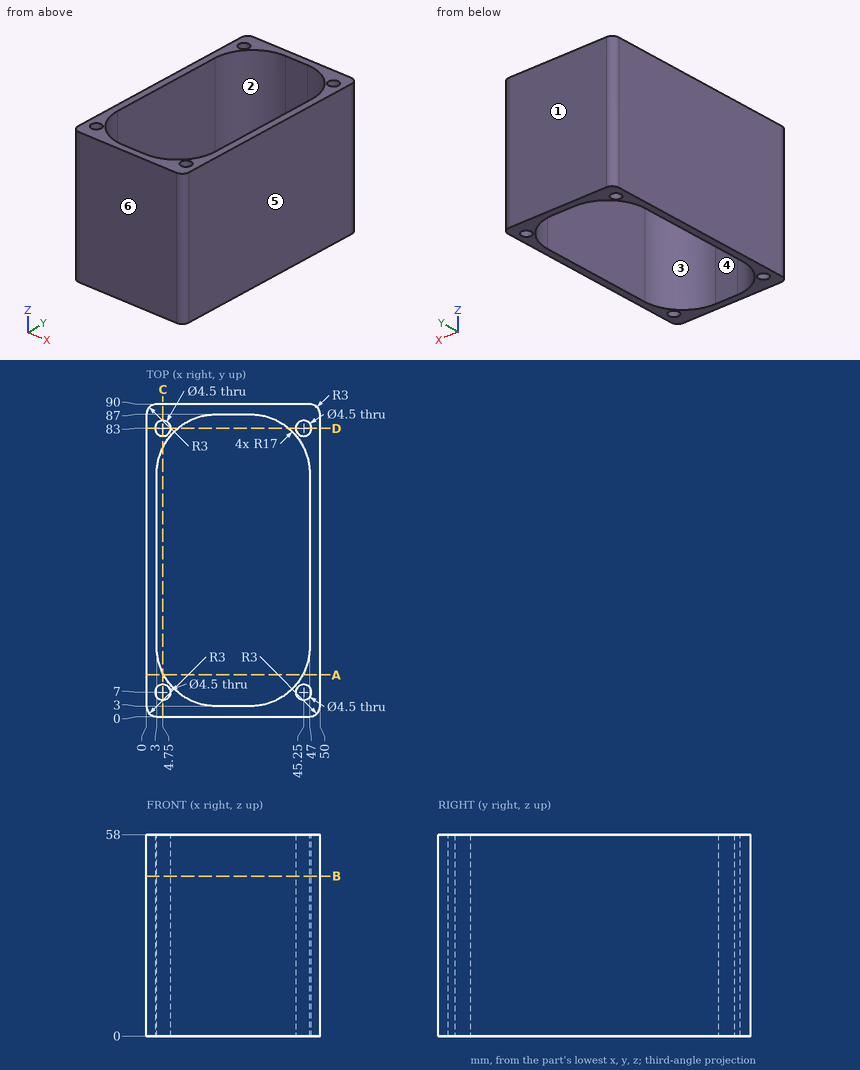
Geometry check sheet. Reference: drawing and pictorial views, mm from the part's lowest x, y, z. A direction names the side the tool comes from. Coordinates: 2 decimals unless noted, no trailing zeros. Order: outer loops, then holes, each group sorted by start corner. A loop starts at its lowest first (then second) coordinate and runs counter-clockwise, first axis right, second up. Notation, with made-up numbers: (63.25, 43) - (85.25, 43) arc R18 cw to (85.25, 66) - close; hole circle Ø9 at (9.5, 29). An arc over 180 degrees is marked (long way). One line per item, written item: value.
(1) Sectioned sample at B-B (z = 46). Enter the section's corners in (x, y), and give its area (3 significant figures).
Data:
outline: (0, 3) arc R3 ccw to (3, 0) - (47, 0) arc R3 ccw to (50, 3) - (50, 87) arc R3 ccw to (47, 90) - (3, 90) arc R3 ccw to (0, 87) - close; hole circle Ø4.5 at (4.75, 7); hole circle Ø4.5 at (4.75, 83); hole (3, 20) arc R17 ccw to (20, 3) - (30, 3) arc R17 ccw to (47, 20) - (47, 70) arc R17 ccw to (30, 87) - (20, 87) arc R17 ccw to (3, 70) - close; hole circle Ø4.5 at (45.25, 7); hole circle Ø4.5 at (45.25, 83)
area: 981 mm^2
(2) Sectioned sample at C-C (x = 4.75). Enter the section's corners in (y, z).
Data:
outline: (0, 0) - (4.75, 0) - (4.75, 58) - (0, 58) - close; (9.25, 0) - (12.49, 0) - (12.49, 58) - (9.25, 58) - close; (77.51, 0) - (80.75, 0) - (80.75, 58) - (77.51, 58) - close; (85.25, 0) - (90, 0) - (90, 58) - (85.25, 58) - close
(3) Release check for a two-part mould opening along Y. For the marked faces 3, 4, 5 and 6 record: +Y half, -Y half, draft (parallel to the pull), parting line (faces both ways), or undercut.
Data:
face 3: undercut
face 4: undercut
face 5: draft
face 6: -Y half
(4) Access from +Z, -Z, +X, -X, +Y, -Y to the whole of each face (thin tool, end or side, straight path). Record for the marked faces 1 and 2.
Data:
face 1: +Z, -Z, +X, -X, +Y
face 2: +Z, -Z
(5) Sectioned sample at A-A (y = 12). Enter the section's corners in (x, z).
Data:
outline: (0, 0) - (5, 0) - (5, 58) - (0, 58) - close; (45, 0) - (50, 0) - (50, 58) - (45, 58) - close
(6) Depth check by flat-ended pin: pin 1 Ø5 at (y, z) = (24, 50.5) entering from -X; pin 2 Ø4 at (x, y) = (8, 77) entering from +Z. Enter the tip coordinate at first touch or a pass-through.
Data:
pin 1: stops at x = 0
pin 2: passes through
(7) Sectioned sample at D-D (y = 83). Enter the section's corners in (x, z), and give its area (3 significant figures).
Data:
outline: (0, 0) - (2.5, 0) - (2.5, 58) - (0, 58) - close; (7, 0) - (9.05, 0) - (9.05, 58) - (7, 58) - close; (40.95, 0) - (43, 0) - (43, 58) - (40.95, 58) - close; (47.5, 0) - (50, 0) - (50, 58) - (47.5, 58) - close
area: 527 mm^2
(8) Thickness scan on probe 1 along X at (y, z) = (57, 18.5); probe 2 along X at (y, z) = (5, 29); probe 3 along Y at (x, z) = (4.75, 33.5). Record the ranges inside material, lowest first. Write a range as from..to.
Data:
probe 1: x = 0..3, 47..50
probe 2: x = 0..3.72, 5.78..12, 38..44.22, 46.28..50
probe 3: y = 0..4.75, 9.25..12.49, 77.51..80.75, 85.25..90
